The figure shows three views and two pictorial views of one solid part (mm, origin at its lowest corner). Answer the questions. A direction names the side the tool comes from. Round coordinates to 2 decimals unless told otherwise and drop trailing zeros. Order: outer loops, then holes, each group sorted by start corner. A loop starts at its lowest first (then second) coordinate and runs counter-clockwise, first axis right, second up. Notation, with made-up numbers: M -30,27.5 L 16,27.5 A27 cw 16,62.5 Z; hole C 55,29.25 d4. An arc over 180 degrees is marked long. Return JSON: item names as keys, results as strings.
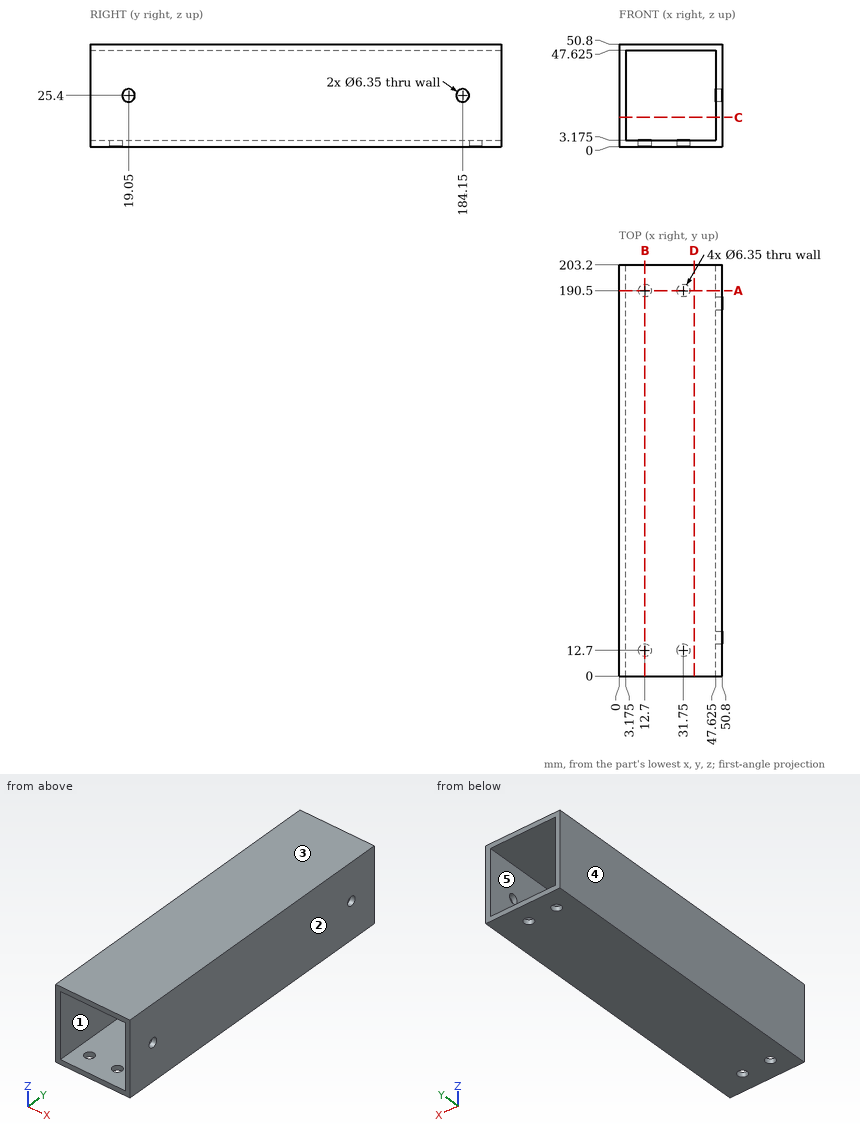
Item 1: Find section B-B (x = 12.7). Determine the outline of the cut face in (y, z) (3 decimals), plus the area to 3 significant figures.
Output:
{"outline": "M 0,0 L 9.525,0 L 9.525,3.175 L 0,3.175 Z; M 0,47.625 L 203.2,47.625 L 203.2,50.8 L 0,50.8 Z; M 15.875,0 L 187.325,0 L 187.325,3.175 L 15.875,3.175 Z; M 193.675,0 L 203.2,0 L 203.2,3.175 L 193.675,3.175 Z", "area": "1,250 mm^2"}
Item 2: Which of the six approach directions +Z, -Z, +X, -X, +Y, -Y give full straight-line access (tool end or side, diameter ignored) to the marked faces 4 and 5?
Output:
{"face 4": "+Z, -Z, -X, +Y, -Y", "face 5": "+Y, -Y"}
Item 3: Consider line 1 along X through (y, z) = (190, 1); line 2 along Y through (x, z) = (50.05, 25.4) (3 decimals); line 3 along Y through (x, z) = (31.75, 2.2) (3 decimals). Determine where each line is inside the solid, lowest interval first. Write a range as [from, to].
Output:
{"line 1": "x = [0, 9.56], [15.84, 28.61], [34.89, 50.8]", "line 2": "y = [0, 15.875], [22.225, 180.975], [187.325, 203.2]", "line 3": "y = [0, 9.525], [15.875, 187.325], [193.675, 203.2]"}
Item 4: The mould has two halves that part along X. Classify the marked faces 1, 2 and 3: pulls with the +X half, pulls with the -X half, needs draft (parallel to the pull), parting line crosses it, or undercut.
Output:
{"face 1": "undercut", "face 2": "pulls with the +X half", "face 3": "needs draft"}
Item 5: Find section C-C (z = 14.5). Determine the outline of the cut face in (x, y) (3 decimals).
Output:
{"outline": "M 0,0 L 3.175,0 L 3.175,203.2 L 0,203.2 Z; M 47.625,0 L 50.8,0 L 50.8,203.2 L 47.625,203.2 Z"}
Item 6: Find section A-A (y = 190.5). Determine the outline of the cut face in (x, z) (3 decimals).
Output:
{"outline": "M 0,0 L 9.525,0 L 9.525,3.175 L 3.175,3.175 L 3.175,47.625 L 47.625,47.625 L 47.625,3.175 L 34.925,3.175 L 34.925,0 L 50.8,0 L 50.8,50.8 L 0,50.8 Z; M 15.875,0 L 28.575,0 L 28.575,3.175 L 15.875,3.175 Z"}
Item 7: Each of these flat-tipped pins is pushed along its axis until it touches: pin 1 (5.5 mm diameter, centred on y = 184.15, z = 25.4, fed in from +X) (3 decimals); pin 2 (4 mm diameter, centred on x = 12.7, y = 12.7, fed in from -Z) (3 decimals). Where does it stop, or does it pass through?
Output:
{"pin 1": "stops at x = 3.175", "pin 2": "stops at z = 47.625"}
Item 8: Find section D-D (x = 37). Determine the outline of the cut face in (y, z) (3 decimals), plus the area to 3 significant figures.
Output:
{"outline": "M 0,0 L 203.2,0 L 203.2,3.175 L 0,3.175 Z; M 0,47.625 L 203.2,47.625 L 203.2,50.8 L 0,50.8 Z", "area": "1,290 mm^2"}
